```python
from build123d import *

# Parameters (mm, degrees)
SKETCH1_W           = 560
SKETCH1_H           = 75
BOSS_EXTRUDE1_DEPTH = 3
SKETCH2_W           = 3
SKETCH2_H           = 10
CUT_EXTRUDE1_DEPTH  = 3
SKETCH3_W           = 3
SKETCH3_H           = 20
SKETCH3_H_2         = 15
CUT_EXTRUDE2_DEPTH  = 3
SKETCH4_W           = 80
SKETCH4_H           = 3
CUT_EXTRUDE3_DEPTH  = 3
SKETCH5_W           = 3
SKETCH5_H           = 14
CUT_EXTRUDE4_DEPTH  = 10


with BuildPart() as part:
    # Sketch1 → Boss-Extrude1 (new body)
    with BuildSketch(Plane.XY):
        with Locations((47.655062333, 176.988975695)):
            Rectangle(SKETCH1_W, SKETCH1_H)
    extrude(amount=BOSS_EXTRUDE1_DEPTH)

    # Sketch2 → Cut-Extrude1 (cut)
    with BuildSketch(Plane.XY.offset(3)):
        with Locations((326.155062333, 189.488975695)):
            Rectangle(SKETCH2_W, SKETCH2_H)
        with Locations((326.155062333, 164.488975695)):
            Rectangle(SKETCH2_W, SKETCH2_H)
    extrude(amount=-CUT_EXTRUDE1_DEPTH, mode=Mode.SUBTRACT)

    # Sketch3 → Cut-Extrude2 (cut)
    with BuildSketch(Plane.XY.offset(3)):
        with Locations((-230.844937667, 204.488975695)):
            Rectangle(SKETCH3_W, SKETCH3_H)
        with Locations((-230.844937667, 149.488975695)):
            Rectangle(SKETCH3_W, SKETCH3_H)
        with Locations((-230.844937667, 176.988975695)):
            Rectangle(SKETCH3_W, SKETCH3_H_2)
    extrude(amount=-CUT_EXTRUDE2_DEPTH, mode=Mode.SUBTRACT)

    # Sketch4 → Cut-Extrude3 (cut)
    with BuildSketch(Plane.XY.offset(3)):
        with Locations((47.655062333, 212.988975695)):
            Rectangle(SKETCH4_W, SKETCH4_H)
    extrude(amount=-CUT_EXTRUDE3_DEPTH, mode=Mode.SUBTRACT)

    # Sketch5 → Cut-Extrude4 (cut)
    with BuildSketch(Plane.XY.offset(3)):
        with Locations((47.655062333, 186.488975695)):
            Rectangle(SKETCH5_W, SKETCH5_H)
        with Locations((47.655062333, 161.488975695)):
            Rectangle(SKETCH5_W, SKETCH5_H)
    extrude(amount=-CUT_EXTRUDE4_DEPTH, mode=Mode.SUBTRACT)


solid = part.part
```
The listing builds one solid part. Answer for the finished solid, in the listing's coordinates (mm). Round coordinates to 2 decimals unless told otherwise and drop trailing zeros. Loops run counter-clockwise (first coordinate to the right, second up) from the corner with the lowest first, then second, coordinate; pieces in that order, holes last.
Q1. Given pin 1 Ø1 at (y, z) = (205.5, 0.5) entering from -X; pin 2 Ø0.9 at (x, z) = (47.5, 1.5) entering from +Y; pin 3 Ø0.9 at (x, z) = (-230.5, 1) entering from +Y, each flat-ended and moving along its own axis, determine where each tip first touches the part or whether it passes through.
Q2. Section A-A, the plane x = 24 is taken. Determine the outline of the cut face in (y, z).
Q3. Find the intervals of material crossed by line 1 (X direction, y = 168, z = 2.05); line 2 (X direction, y = 195, z = 1.2); line 3 (X direction, y = 181.5, z = 1.7), in increasing order.
Completed:
1. pin 1: stops at x = -229.34
1. pin 2: stops at y = 211.49
1. pin 3: stops at y = 194.49
2. outline: (139.49, 0) - (211.49, 0) - (211.49, 3) - (139.49, 3) - close
3. line 1: x = -232.34 to 46.16, 49.16 to 324.66
3. line 2: x = -229.34 to 327.66
3. line 3: x = -229.34 to 46.16, 49.16 to 327.66
